Read the model definition and answer for the solid it produces. Units are mm, in the model's axes. Face numbers are marked on the shaded views. A direction names the side the tool comes from. Give positions to 0.01 mm unless a question says otherwise; leave off trailing zeros. Order: outer loops, then holes, each group sorted by start corner. A loop starts at its lowest first (then second) coordinate and runs counter-clockwise, first axis right, second up.
Item 1: A cutting plane is placed at B-B (z = -11). Write down the section's boundary in (x, y), plus the area to 3 significant figures.
Item 2: A cutting plane is placed at A-A (z = 10). Write down the section's boundary in (x, y) (3 decimals), plus the area to 3 significant figures.
Item 3: A cutting plane is placed at C-C (x = -5.25). Write down the section's boundary in (y, z).
Item 4: Given pin 1 Ø1.5 at (x, y) = (5, 4) entering from -Z; pin 2 Ø1.2 at (x, z) = (-3.35, -11) entering from +Y; pin 3 Ø1.6 at (y, z) = (0.5, 2) entering from -X, each flat-ended and moving along its own axis, determine where each tip first touches the part or whether it passes through.
Item 5: Find the intervals of material crossed by line 1 along X through (y, z) = (8.7, -11); line 2 along Y through (x, z) = (2.5, -6.5); line 3 along Z through (x, y) = (-4.5, 1.5), in increasing order.
Item 6: A cutting plane is placed at D-D (x = 3.15). Write down the section's boundary in (y, z).
Item 7: The mould has two halves that part along Y. Classify the marked faces 1, 2 and 3: +Y half, -Y half, draft (parallel to the pull), parting line (faces both ways), or undercut.
Item 8: Which of the six approach directions +Z, -Z, +X, -X, +Y, -Y give full straight-line access (tool end or side, diameter ignored) to the marked faces 4, 5 and 6?
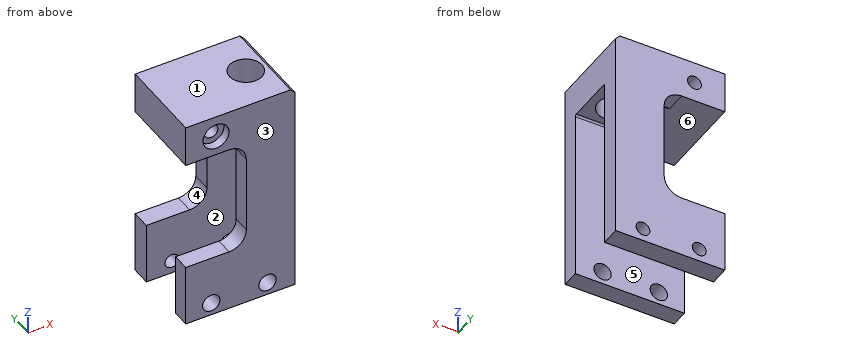
from build123d import *

# Parameters (mm, degrees)
SKETCH1_W                   = 12.6
SKETCH1_H                   = 25
BOSS_EXTRUDE1_DEPTH         = 10
CUT_EXTRUDE1_START          = -4.8
SKETCH2_W                   = 7
SKETCH2_H                   = 5.8
CUT_EXTRUDE1_DEPTH          = 23.853028767
SKETCH3_W                   = 20.2
SKETCH3_H                   = 5.8
CUT_EXTRUDE2_DEPTH          = 18.47140521
SKETCH6_R                   = 1
CUT_EXTRUDE5_DEPTH          = 17.122654868
TAP_DRILL_FOR_M2X0_4_TAP1_D = 1.6
CUT_EXTRUDE6_DEPTH          = 17.122654868
CUT_EXTRUDE6_DEPTH_BACK     = 17.122654868
SKETCH9_W                   = 7
SKETCH9_H                   = 13
FILLET1_R                   = 2
SKETCH4_R                   = 1.875
CUT_EXTRUDE7_DEPTH          = 24.403632197
TAP_DRILL_FOR_M2X0_4_TAP4_D = 1.6
FILLET3_R                   = 0.2
CHAMFER2_SIZE               = 0.5
SKETCH25_R                  = 1.5
CUT_EXTRUDE19_DEPTH         = 1


with BuildPart() as part:
    # Sketch1 → Boss-Extrude1 (new body)
    with BuildSketch(Plane(origin=(0, 0, 0), x_dir=(1, 0, 0), z_dir=(0, 1, 0))):
        Rectangle(SKETCH1_W, SKETCH1_H)
    extrude(amount=BOSS_EXTRUDE1_DEPTH)

    # Sketch2 → Cut-Extrude1 (cut, through all)
    with BuildSketch(Plane.XY.offset(12.5).offset(CUT_EXTRUDE1_START)):
        with Locations((-2.8, 4.9)):
            Rectangle(SKETCH2_W, SKETCH2_H)
    extrude(amount=-CUT_EXTRUDE1_DEPTH, mode=Mode.SUBTRACT)

    # Sketch3 → Cut-Extrude2 (cut, through all)
    with BuildSketch(Plane.ZY.offset(-0.7)):
        with Locations((-2.4, 4.9)):
            Rectangle(SKETCH3_W, SKETCH3_H)
    extrude(amount=-CUT_EXTRUDE2_DEPTH, mode=Mode.SUBTRACT)

    # Sketch6 → Cut-Extrude5 (cut, through all)
    with BuildSketch(Plane(origin=(0, 2, 0), x_dir=(1, 0, 0), z_dir=(0, 1, 0))):
        with Locations(Location((3.15, 11, 0), (0, 0, 270))):
            Circle(SKETCH6_R)
        with Locations(Location((-3.35, 11, 0), (0, 0, 270))):
            Circle(SKETCH6_R)
    extrude(amount=-CUT_EXTRUDE5_DEPTH, mode=Mode.SUBTRACT)

    # Tap Drill for M2x0.4 Tap1 (through all)
    with Locations(Plane(origin=(3.15, 10, -11), x_dir=(0, 0, 1), z_dir=(0, 1, 0))):
        with Locations((0, 0), (0, -6.5)):
            Hole(TAP_DRILL_FOR_M2X0_4_TAP1_D / 2)

    # Sketch9 → Cut-Extrude6 (cut, two sides: drawn at the far end of the back side and taken through both)
    with BuildSketch(Plane(origin=(0, 2, 0), x_dir=(1, 0, 0), z_dir=(0, 1, 0)).offset(-CUT_EXTRUDE6_DEPTH_BACK)):
        with Locations((-2.8, -1.2)):
            Rectangle(SKETCH9_W, SKETCH9_H)
    extrude(amount=CUT_EXTRUDE6_DEPTH + CUT_EXTRUDE6_DEPTH_BACK, mode=Mode.SUBTRACT)

    # Fillet1
    fillet1_edges = [part.edges().sort_by_distance(p)[0] for p in [
        (0.7, 8.9, 7.7),
        (0.7, 1, 7.7),
        (0.7, 8.9, -5.3),
        (0.7, 1, -5.3),
    ]]
    fillet(fillet1_edges, radius=FILLET1_R)

    # Sketch4 → Cut-Extrude7 (cut, through all)
    with BuildSketch(Plane(origin=(0, 0, 7.7), x_dir=(-1, 0, 0), z_dir=(0, 0, -1))):
        with Locations((-3.5, 4.9)):
            Circle(SKETCH4_R)
    extrude(amount=-CUT_EXTRUDE7_DEPTH, mode=Mode.SUBTRACT)

    # Tap Drill for M2x0.4 Tap4 (through all)
    with Locations(Plane(origin=(-2.8, 10, 10), x_dir=(0, 0, 1), z_dir=(0, 1, 0))):
        with Locations((0, 0)):
            Hole(TAP_DRILL_FOR_M2X0_4_TAP4_D / 2)

    # Fillet3
    fillet3_edges = [part.edges().sort_by_distance(p)[0] for p in [
        (2.5, 7.8, 7.7),
        (2.5, 2, 7.7),
    ]]
    fillet(fillet3_edges, radius=FILLET3_R)

    # Chamfer2
    chamfer2_edges = [part.edges().sort_by_distance(p)[0] for p in [
        (6.3, 5, 12.5),
    ]]
    chamfer(chamfer2_edges, length=CHAMFER2_SIZE)

    # Sketch25 → Cut-Extrude19 (cut)
    with BuildSketch(Plane.XZ):
        with Locations(Location((-2.8, 10, 0), (0, 0, 270))):
            Circle(SKETCH25_R)
    extrude(amount=-CUT_EXTRUDE19_DEPTH, mode=Mode.SUBTRACT)


solid = part.part
Response values:
1. outline: (-6.3, 0) - (-4.35, 0) - (-4.35, 2) - (-6.3, 2) - close; (-6.3, 7.8) - (-4.15, 7.8) - (-4.15, 10) - (-6.3, 10) - close; (-2.55, 7.8) - (2.35, 7.8) - (2.35, 10) - (-2.55, 10) - close; (-2.35, 0) - (2.15, 0) - (2.15, 2) - (-2.35, 2) - close; (3.95, 7.8) - (6.3, 7.8) - (6.3, 10) - (3.95, 10) - close; (4.15, 0) - (6.3, 0) - (6.3, 2) - (4.15, 2) - close
1. area: 37.9 mm2
2. outline: (-6.3, 0) - (-4.3, 0) - (-4.3, 1) - (-3.6, 1) - (-3.6, 10) - (-6.3, 10) - close; (-2, 1) - (-1.3, 1) - (-1.3, 0) - (6.3, 0) - (6.3, 10) - (-2, 10) - close; hole circle Ø3.75 at (3.5, 4.9)
2. area: 97.6 mm2
3. outline: (0, -12.5) - (2, -12.5) - (2, -5.3) - (0, -5.3) - close; (0, 7.7) - (10, 7.7) - (10, 12.5) - (0, 12.5) - close; (7.8, -12.5) - (10, -12.5) - (10, -5.3) - (7.8, -5.3) - close
4. pin 1: stops at z = 7.7
4. pin 2: passes through
4. pin 3: stops at x = 0.7
5. line 1: x = -6.3 to -4.15, -2.55 to 2.35, 3.95 to 6.3
5. line 2: y = 0 to 2, 7.8 to 10
5. line 3: z = -12.5 to -5.3, 7.7 to 12.5
6. outline: (0, -12.5) - (2, -12.5) - (2, -12) - (0, -12) - close; (0, -10) - (2, -10) - (2, 7.5) arc R0.2 cw to (2.2, 7.7) - (3.06, 7.7) - (3.06, 12.5) - (0, 12.5) - close; (6.74, 7.7) - (7.6, 7.7) arc R0.2 cw to (7.8, 7.5) - (7.8, -10.2) - (10, -10.2) - (10, 12.5) - (6.74, 12.5) - close; (7.8, -12.5) - (10, -12.5) - (10, -11.8) - (7.8, -11.8) - close
7. face 1: draft
7. face 2: undercut
7. face 3: -Y half
8. face 4: -X, +Y, -Y
8. face 5: -Z, +X, -X
8. face 6: -X
